```python
from build123d import *

# Parameters (mm, degrees)
SKETCH1_R           = 0.5
SKETCH1_W           = 3
SKETCH1_H           = 3
BOSS_EXTRUDE1_DEPTH = 4
SKETCH_1_R          = 0.5
CUT_EXTRUDE_1_DEPTH = 12


with BuildPart() as part:
    # Sketch1 → Boss-Extrude1 (new body)
    with BuildSketch(Plane.XY):
        Polygon((3.5, -3.5), (-3.5, -3.5), (-3.5, 3.5), (-3.5, 19.763228949), (-5.5, 19.763228949), (-5.5, 24.763228949), (-3.5, 24.763228949), (-3.5, 27.5), (-3.5, 29.5), (3.5, 29.5), (3.5, 27.5), (3.5, 24.763228949), (5.5, 24.763228949), (5.5, 19.763228949), (3.5, 19.763228949), (3.5, 3.5), align=None)
        with Locations((-1.2, 28.5)):
            Circle(SKETCH1_R, mode=Mode.SUBTRACT)
        with Locations((1.2, 28.5)):
            Circle(SKETCH1_R, mode=Mode.SUBTRACT)
        Polygon((2, 4.263228949), (-2, 4.263228949), (-2, 21.263228949), (-4, 21.263228949), (-4, 23.263228949), (-2, 23.263228949), (-2, 27.5), (2, 27.5), (2, 23.263228949), (4, 23.263228949), (4, 21.263228949), (2, 21.263228949), align=None, mode=Mode.SUBTRACT)
        Rectangle(SKETCH1_W, SKETCH1_H, mode=Mode.SUBTRACT)
    extrude(amount=BOSS_EXTRUDE1_DEPTH)

    # 草图1 → 切除-拉伸1 (cut, through all)
    with BuildSketch(Plane.ZY.offset(5.5)):
        with Locations((2, 22.263228949)):
            Circle(SKETCH_1_R)
    extrude(amount=-CUT_EXTRUDE_1_DEPTH, mode=Mode.SUBTRACT)


solid = part.part
```
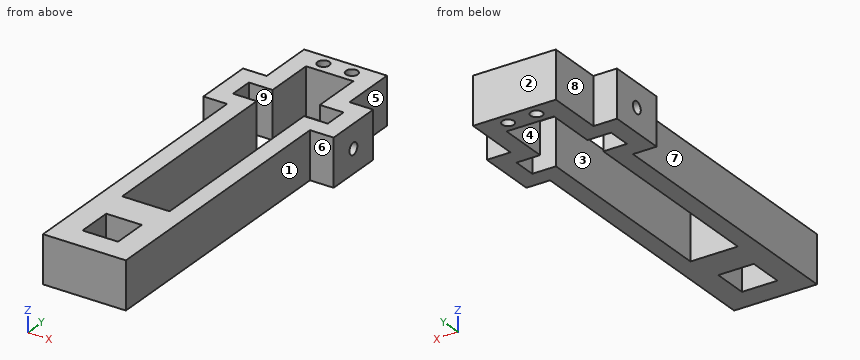
Build history of the part. All positions in model axes, mm. Face numbers are marked on the shaded views. A direction names the side the tool comes from. Give positions to 0.01 mm unless a question says otherwise; leave off trailing zeros. Loops run counter-clockwise (first coordinate to the right, second up) from the corner with the lowest first, then second, coordinate; pieces in that order, holes last. Notation, with made-up numbers: (79, 60.5) -> (107, 60.5) arc R12 cw to (107, 81.5) -> close; hole circle Ø3 at (38, -10). An arc over 180 degrees is marked (long way). One line per question, with ' | ' between items. Start each with the question number.
1) Cut at D-D (x = -2.5). Give the cut face in (y, z).
2) Two-plate mould, pull along Y, no slides. Class the marked faces 1, 2, 3 and 4: released by +Y, released by -Y, zero draft, split by the parting line, or undercut.
3) 3-axis set-ups, long thin cutter, end or side, ignore diameter. For the marked faces 5, 6, 7, 8 and 9: which of +Z, -Z, +X, -X, +Y, -Y reach the whole face in a straight line?
4) Cut at B-B (z = 2.9). Count the separate pieces of the cut face and the enclosed holes in it, plus the area to 3 significant figures.
5) Cut at C-C (y = 28.5). Give the cut face in (x, z).
6) Pin check, flat tips, straight feed: pin 1 (1.2 mm diameter, centred on y = 26.5, z = 2, fed in from -X); pin 2 (2 mm diameter, centred on x = 5, z = 3, fed in from +Y). Stop position of each tip, or through.
7) Probe L1, parallel to Y at x = 0.5, z = 1.55; L2, parallel to Y at x = -1.2, z = 1.8; L3, parallel to Y at x = 4.4, z = 2. List the from-to ranges inside material, lowest first.
8) Cut at A-A (x = -1.2). Give the cut face in (y, z), plus the area to 3 significant figures.
Return value:
1) outline: (-3.5, 0) -> (21.26, 0) -> (21.26, 4) -> (-3.5, 4) -> close; (23.26, 0) -> (29.5, 0) -> (29.5, 4) -> (23.26, 4) -> close
2) face 1: zero draft | face 2: released by +Y | face 3: undercut | face 4: undercut
3) face 5: +Z, -Z, +X, +Y | face 6: +Z, -Z, +X, -Y | face 7: +Z, -Z, -X, -Y | face 8: +Z, -Z, -X, +Y | face 9: +Z, -Z
4) separate pieces: 1 | enclosed holes: 4 | area: 139 mm^2
5) outline: (-3.5, 0) -> (-1.7, 0) -> (-1.7, 4) -> (-3.5, 4) -> close; (-0.7, 0) -> (0.7, 0) -> (0.7, 4) -> (-0.7, 4) -> close; (1.7, 0) -> (3.5, 0) -> (3.5, 4) -> (1.7, 4) -> close
6) pin 1: x = -3.5 | pin 2: y = 24.76
7) L1: -3.5 to -1.5, 1.5 to 4.26, 27.5 to 29.5 | L2: -3.5 to -1.5, 1.5 to 4.26, 27.5 to 28, 29 to 29.5 | L3: 19.76 to 21.76, 22.76 to 24.76
8) outline: (-3.5, 0) -> (-1.5, 0) -> (-1.5, 4) -> (-3.5, 4) -> close; (1.5, 0) -> (4.26, 0) -> (4.26, 4) -> (1.5, 4) -> close; (27.5, 0) -> (28, 0) -> (28, 4) -> (27.5, 4) -> close; (29, 0) -> (29.5, 0) -> (29.5, 4) -> (29, 4) -> close | area: 23.1 mm^2
